Source: CAD feature listing. Evaluate the final solid. Frame: model axes, mm. A direction names the side the tool comes from. Give positions to 0.01 mm unless a question says otherwise; leave off trailing zeros. Write each loop counter-clockwise with the first axis right and the second up, starting at its lowest first coordinate (ties: lowest second). Pieces come first, ordered by that corner, then holes.
```python
from build123d import *

# Parameters (mm, degrees)
F1_W     = 28.5
F1_H     = 144.5
F1_W_2   = 26.9
F1_H_2   = 142.9
F2_DEPTH = 0.5
F3_DEPTH = 15
F4_SIZE2 = 14
F4_SIZE  = 3
F5_R     = 0.8
F7_DEPTH = 10


with BuildPart() as f2:
    # F1 (on Top) → F2 (new body)
    with BuildSketch(Plane.XY):
        Rectangle(F1_W, F1_H)
        Rectangle(F1_W_2, F1_H_2, mode=Mode.SUBTRACT)
    extrude(amount=F2_DEPTH)

    # F1 (on Top) → F3 (join)
    with BuildSketch(Plane.XY):
        Rectangle(F1_W, F1_H)
        Rectangle(F1_W_2, F1_H_2, mode=Mode.SUBTRACT)
        Rectangle(F1_W_2, F1_H_2)
    extrude(amount=-F3_DEPTH)

    # F4
    f4_edges = [f2.edges().sort_by_distance(p)[0] for p in [
        (0, -72.25, -15),
        (14.25, 0, -15),
        (0, 72.25, -15),
        (-14.25, 0, -15),
    ]]
    f4_side = f2.faces().sort_by_distance((0, 0, -15))[0]
    chamfer(f4_edges, length=F4_SIZE, length2=F4_SIZE2, reference=f4_side)

    # F5
    f5_edges = [f2.edges().sort_by_distance(p)[0] for p in [
        (12.75, 70.75, -8),
        (-12.75, 70.75, -8),
        (12.75, -70.75, -8),
        (-12.75, -70.75, -8),
    ]]
    fillet(f5_edges, radius=F5_R)

    # F6 (on face) → F7 (cut)
    with BuildSketch(Plane(origin=(0, 0, -15), x_dir=(1, 0, 0), z_dir=(0, 0, -1))):
        Polygon((-8.55, 39.1863448016), (-8.55, 29.3136551984), (0, 24.3773103969), (8.55, 29.3136551984), (8.55, 39.1863448016), (0, 44.1226896031), align=None)
        Polygon((-8.55, -39.1863448016), (0, -44.1226896031), (8.55, -39.1863448016), (8.55, -29.3136551984), (0, -24.3773103969), (-8.55, -29.3136551984), align=None)
    extrude(amount=-F7_DEPTH, mode=Mode.SUBTRACT)


solid = f2.part
```
1. Access query for faces 4 (the flat face through (-8.55, 34, -10)), 5 (the flat face through (12.77, -1, -7.9)). Directions: +Z, -Z, +X, -X, +Y, -Y. A direction counts if a zero-diameter tool reaches every point of the face in a straight line with its end or side. Return the directions, or none.
2. Section query A-A (y = -3). Return loops of the section in (x, z).
3. Section query C-C (z = -7.5). Give the number of separate pieces and of enclosed holes in the cut face, plus the area to 3 significant figures.
4. Section query B-B (x = 4). Return loops of the section in (y, z).
5. Pin query (flat end, axial travel): P1, Ø3, axis at x = 1, y = -49.5, coming from the +Z side; P2, Ø2, axis at y = 47.5, z = -9, coming from the -X side; P3, Ø5, axis at y = 34.5, z = -8, coming from the +X side. Return the tip coordinate at first contact, or that it passes through.
6. Line query: probe 1 along Z at (x, y) = (-10.5, 16); probe 2 along Y at (x, z) = (-5.25, -6); probe 3 along Z at (x, y) = (2.5, -26.5). Output: solid intervals per line, ascending.
7. Pull-direction query (Y, two-part tool) for faces 1 (the flat face through (0, 1, 0)), 2 (the cylindrical face through (12.6, -70.7, -7.4)), 3 (the flat face through (-0.19, 70.77, -7.9)); classes: pulls with the +Y half, pulls with the -Y half, needs draft (parallel to the pull), parting line crosses it, or undercut.
8. Section query D-D (y = 33). Return loops of the section in (x, z).
The answers:
1. face 4: -Z
1. face 5: -Z, +X, +Y, -Y
2. outline: (-14.25, -1) - (-11.25, -15) - (11.25, -15) - (14.25, -1) - (14.25, 0.5) - (13.45, 0.5) - (13.45, 0) - (-13.45, 0) - (-13.45, 0.5) - (-14.25, 0.5) - close
3. separate pieces: 1
3. enclosed holes: 2
3. area: 3,140 mm2
4. outline: (-72.25, -1) - (-69.25, -15) - (-41.81, -15) - (-41.81, -5) - (-26.69, -5) - (-26.69, -15) - (26.69, -15) - (26.69, -5) - (41.81, -5) - (41.81, -15) - (69.25, -15) - (72.25, -1) - (72.25, 0.5) - (71.45, 0.5) - (71.45, 0) - (-71.45, 0) - (-71.45, 0.5) - (-72.25, 0.5) - close
5. P1: stops at z = 0
5. P2: stops at x = -12.75
5. P3: stops at x = 13.29
6. probe 1: z = -15 to 0
6. probe 2: y = -71.18 to -41.09, -27.41 to 27.41, 41.09 to 71.18
6. probe 3: z = -5 to 0
7. face 1: undercut
7. face 2: pulls with the -Y half
7. face 3: pulls with the +Y half
8. outline: (-14.25, -1) - (-11.25, -15) - (-8.55, -15) - (-8.55, -5) - (8.55, -5) - (8.55, -15) - (11.25, -15) - (14.25, -1) - (14.25, 0.5) - (13.45, 0.5) - (13.45, 0) - (-13.45, 0) - (-13.45, 0.5) - (-14.25, 0.5) - close
